The model under review builds one solid part; all positions refer to its coordinate system, in mm. A direction names the side the tool comes from. Coordinates: 2 decimals unless noted, no trailing zeros. Write each loop counter-clockwise with the first axis right and the second up, starting at its lowest first coordinate (ties: lowest second). Pieces come first, ordered by that corner, then holes. Notation, with made-up numbers: (53, -15) -> (83, -15) arc R16 cw to (83, 5) -> close; hole circle Ø11 at (11, 10.25). An arc over 180 degrees is marked (long way). Write each question's results on one line, items separated by ' | '.
```python
from build123d import *

# Parameters (mm, degrees)
EXTRUDE_1_DEPTH      = 10
EXTRUDE_2_DEPTH      = 68
SKETCH_9_W           = 24
SKETCH_9_H           = 50
EXTRUDE_4_DEPTH      = 20
SKETCH_10_R          = 13
CUT_EXTRUDE_3_DEPTH  = 109.53570841
FILLET_6_R           = 25
SKETCH_22_W          = 24
SKETCH_22_H          = 5
EXTRUDE_5_DEPTH      = 10
M8X1_0_1_D           = 7
M8X1_0_1_CSINK_D     = 8.05
M8X1_0_1_CSINK_ANGLE = 90


with BuildPart() as part:
    # 草图1 → 凸台-拉伸1 (new body)
    with BuildSketch(Plane(origin=(0, 0, 0), x_dir=(1, 0, 0), z_dir=(0, 1, 0))):
        Polygon((12, 37.5), (12, 40), (-12, 40), (-12, 37.5), (-12, -37.5), (-12, -40), (12, -40), (12, -37.5), align=None)
    extrude(amount=EXTRUDE_1_DEPTH)

    # 草图2 → 凸台-拉伸2 (add)
    with BuildSketch(Plane(origin=(0, 10, 0), x_dir=(1, 0, 0), z_dir=(0, 1, 0))):
        Polygon((-4, 25), (-12, 25), (-12, -25), (-4, -25), (4, -25), (12, -25), (12, 25), (4, 25), align=None)
    extrude(amount=EXTRUDE_2_DEPTH)

    # 草图9 → 凸台-拉伸4 (add)
    with BuildSketch(Plane(origin=(0, 78, 0), x_dir=(1, 0, 0), z_dir=(0, 1, 0))):
        Rectangle(SKETCH_9_W, SKETCH_9_H)
    extrude(amount=EXTRUDE_4_DEPTH)

    # 草图10 → 切除-拉伸3 (cut, through all)
    with BuildSketch(Plane.ZY.offset(12)):
        with Locations((0, 78)):
            Circle(SKETCH_10_R)
    extrude(amount=-CUT_EXTRUDE_3_DEPTH, mode=Mode.SUBTRACT)

    # 圆角6
    fillet_6_edges = [part.edges().sort_by_distance(p)[0] for p in [
        (0, 98, -25),
        (0, 98, 25),
    ]]
    fillet(fillet_6_edges, radius=FILLET_6_R - 0.0001)  # a hair under: the kernel refuses the full size

    # 草图22 → 凸台-拉伸5 (add)
    with BuildSketch(Plane.XZ):
        with Locations((0, 42.5)):
            Rectangle(SKETCH_22_W, SKETCH_22_H)
        with Locations((0, -42.5)):
            Rectangle(SKETCH_22_W, SKETCH_22_H)
    extrude(amount=-EXTRUDE_5_DEPTH)

    # M8x1.0 螺纹孔1 (through all)
    with Locations(Plane(origin=(0, 10, 0), x_dir=(1, 0, 0), z_dir=(0, 1, 0))):
        with Locations((0, -35), (0, 35)):
            CounterSinkHole(M8X1_0_1_D / 2, M8X1_0_1_CSINK_D / 2, counter_sink_angle=M8X1_0_1_CSINK_ANGLE)


solid = part.part
```
Q1. Machinability: for faces 4 (the flat face through (-0.2, 10, 30.7)), 5 (the flat face through (0, 0, 1)), 6 (the flat face through (0, 41, -25)), which of the approach directions +Z, -Z, +X, -X, +Y, -Y give a long, thin tool a straight path to every point of the face, cutting with its end or side? Answer none if there is none.
Solution:
face 4: +Z, +X, -X, +Y | face 5: +Z, -Z, +X, -X, -Y | face 6: -Z, +X, -X, +Y
Q2. Draft analysis for pull direction Z (two halves, no side actions). For faces 1 (the flat face through (0, 41, 25)), 2 (the cylindrical face through (-0.17, 65.31, -2.82)), 3 (the flat face through (0, 5, -45)), state which applies: pulls with the +Z half, pulls with the -Z half, needs draft (parallel to the pull), parting line crosses it, or undercut.
Solution:
face 1: pulls with the +Z half | face 2: undercut | face 3: pulls with the -Z half
Q3. Add section B-B (x = 0). Count the separate pieces of the cut face and the enclosed holes in it, plus the area to 3 significant figures.
Solution:
separate pieces: 3 | enclosed holes: 1 | area: 4,360 mm²
Q4. Add section D-D (y = 33.5). Write out the cut boundary in (x, z), plus the area to 3 significant figures.
Solution:
outline: (-12, -25) -> (12, -25) -> (12, 25) -> (-12, 25) -> close | area: 1,200 mm²
Q5. Add section A-A (z = 35). Write out the cut boundary in (x, y) (3 decimals).
Solution:
outline: (-12, 0) -> (-3.5, 0) -> (-3.5, 9.475) -> (-4.025, 10) -> (-12, 10) -> close; (3.5, 0) -> (12, 0) -> (12, 10) -> (4.025, 10) -> (3.5, 9.475) -> close
Q6. For line 1 (Z direction, x = 0, y = 7.25); line 2 (Y direction, x = -2.25, z = -0.5) (3 decimals); line 3 (X direction, y = 3, z = -35), list the stretches that pass through material, from the lowest coordinate up. Write a range as from..to.
Solution:
line 1: -45..-38.5, -31.5..31.5, 38.5..45 | line 2: 0..65.01, 90.99..97.995 | line 3: -12..-3.5, 3.5..12
Q7. Clearance check with flat-ended pins moving along their axes: P1, Ø10, axis at x = 1, z = 39.5, coming from the +Y side; P2, Ø21, axis at y = 78, z = 0, coming from the -X side; P3, Ø2, axis at x = 7, y = 47, coming from the +Z side; P4, Ø8, axis at x = 9, z = 14, coming from the +Y side. State where each tip first meets the part, or that it passes through.
Solution:
P1: y = 10 | P2: through | P3: z = 25 | P4: y = 95.91
